from build123d import *

# Parameters (mm, degrees)
F0_R     = 38.5
F0_R_2   = 36.5
F1_DEPTH = 10
F2_R     = 42
F3_DEPTH = 8
F4_SIZE  = 7


with BuildPart() as f1:
    # F0 (on Top) → F1 (new body)
    with BuildSketch(Plane.XY):
        Circle(F0_R)
        Circle(F0_R_2, mode=Mode.SUBTRACT)
    extrude(amount=F1_DEPTH)

    # F2 (on Top) → F3 (join)
    with BuildSketch(Plane.XY):
        Circle(F2_R)
    extrude(amount=-F3_DEPTH)

    # F4
    f4_edges = [f1.edges().sort_by_distance(p)[0] for p in [
        (-42, 0, -8),
    ]]
    chamfer(f4_edges, length=F4_SIZE)


solid = f1.part
Input: part model. Units: mm. Frame: model coordinates. A direction names the side the tool comes from. Give positions to 0.01 mm unless a question says otherwise; leave off trailing zeros. Write each loop counter-clockwise with the first axis right and the second up, starting at its lowest first coordinate (ties: lowest second). Pieces come first, ordered by that corner, then holes.
Q1. First-contact query: P1, Ø10, axis at x = 33, y = -32, coming from the -Z side; P2, Ø1, axis at x = -15, y = -21, coming from the +Z side; P3, Ø1, axis at x = 15, z = -4.5, coming from the -Y side. Flat tips, straight axial feed; report the tip coordinate or a pass-through.
Q2. Section D-D, the plane z = -4.25. Output: boundary loops of the cut face in (x, y), plus the area to 3 significant figures.
Q3. Pull-direction query (X, two-part tool) for faces 1 (the face through (23, 29, 10)), 2 (the face through (-7.912, -35.632, 4.93)), 3 (the face through (-1, 1, 0)), 4 (the face through (-28, -21.5, -7.7)); classes: pulls with the +X half, pulls with the -X half, needs draft (parallel to the pull), parting line crosses it, or undercut.
Q4. Set-up query: faces 5 (the face through (40.06, 12.62, -0.49)), 6 (the face through (18.5, -34, 0)). Return all of +Z, -Z, +X, -X, +Y, -Y with unobstructed straight access to the full face (end or side cutting, diameter ignored); none if empty.
Q5. Material intervals for probe 1 along Y at (x, z) = (0, 8); probe 2 along Z at (x, y) = (1, 13); probe 3 along Y at (x, z) = (-16.5, 4.25), sorted ascending.
Q6. Section A-A, the plane y = 0. Output: boundary loops of the cut face in (x, z).
Q7. Section C-C, the plane z = 6. Output: boundary loops of the cut face in (x, y).
Filled in:
1. P1: stops at z = -2.03
1. P2: stops at z = 0
1. P3: stops at y = -36.04
2. outline: circle Ø77.5 at (0, 0)
2. area: 4,720 mm2
3. face 1: needs draft
3. face 2: undercut
3. face 3: undercut
3. face 4: parting line crosses it
4. face 5: +Z, -Z
4. face 6: +Z
5. probe 1: y = -38.5 to -36.5, 36.5 to 38.5
5. probe 2: z = -8 to 0
5. probe 3: y = -34.79 to -32.56, 32.56 to 34.79
6. outline: (-42, -1) - (-35, -8) - (35, -8) - (42, -1) - (42, 0) - (38.5, 0) - (38.5, 10) - (36.5, 10) - (36.5, 0) - (-36.5, 0) - (-36.5, 10) - (-38.5, 10) - (-38.5, 0) - (-42, 0) - close
7. outline: circle Ø77 at (0, 0); hole circle Ø73 at (0, 0)
